Part print with two shaded views. Sizes in mm from the minimum x, y, z corner. A direction names the side the tool comes from. Give positions to 0.01 mm unless a question says otherwise; leave off trailing zeros. Write each loop counter-clockwise with the first axis right and the second up, starting at its lowest first coordinate (ties: lowest second). Pieces come first, ordered by that corner, then holes. Notation, with made-up numbers: M -26.5,17.5 L 6.5,17.5 A33 cw 6.5,56.5 Z; hole C 78,30.25 d1. An arc over 180 degrees is marked long. Return JSON: item names as keys, results as strings. Group by question number.
Q1. Pull direction X, two halves, no side cores. Call the marked faces 1, 2, 3 and 4: +X half, -X half, draft (parallel to the pull), parting line (faces both ways), or undercut.
Q2. Flat gauge pins, fed straight in: pin 1 Ø9.5 at (x, y) = (13.5, 15.5) entering from -Z; pin 2 Ø2 at (x, z) = (12, 21) entering from +Y. Where does each tip first touch, or does it go through?
Q3. Band-saw the part on A-A, the plane z = 5. Give the cut face in (x, y).
Q4. Wall check: probe 1 along Z at (x, y) = (15.25, 3); probe 2 along X at (y, z) = (4.75, 23.5). Give the ranges that are in metal, low to high.
Q5. Tool access for the marked faces 5 and 6: list every direction of +Z, -Z, +X, -X, +Y, -Y with a clear straight run to the whole face (end or side of a thin tool).
Q6. Band-saw the part on C-C, the plane y = 9.25. Give the cut face in (x, z) (3 decimals).
Q7. Band-saw the part on B-B, the plane x = 18.25. Give the cut face in (y, z), then the cut area to 3 significant figures.
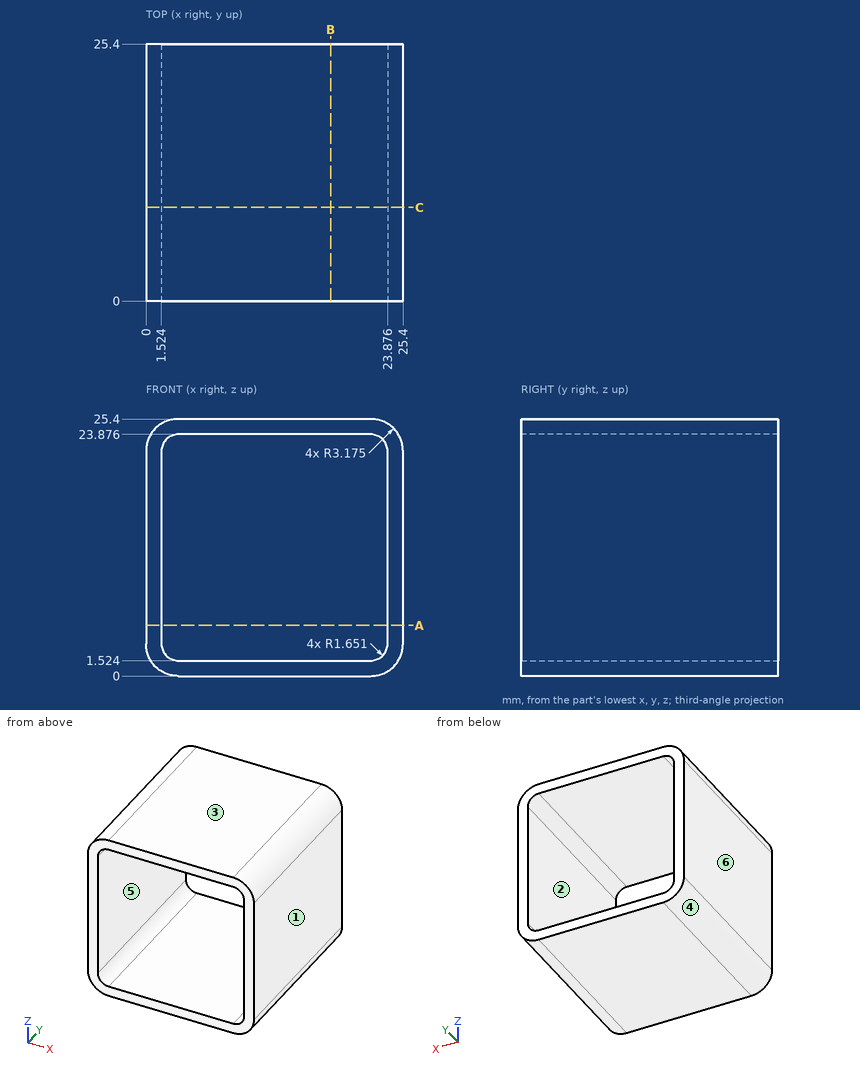
From the geometry:
{
 "1": {"face 1": "+X half", "face 2": "undercut", "face 3": "draft", "face 4": "-X half"},
 "2": {"pin 1": "stops at z = 0", "pin 2": "passes through"},
 "3": {"outline": "M 0,0 L 1.52,0 L 1.52,25.4 L 0,25.4 Z; M 23.88,0 L 25.4,0 L 25.4,25.4 L 23.88,25.4 Z"},
 "4": {"probe 1": "z = 0 to 1.52, 23.88 to 25.4", "probe 2": "x = 0.27 to 2.13, 23.27 to 25.13"},
 "5": {"face 5": "+Y, -Y", "face 6": "+Z, -Z, -X, +Y, -Y"},
 "6": {"outline": "M 0,3.175 A3.175 ccw 3.175,0 L 22.225,0 A3.175 ccw 25.4,3.175 L 25.4,22.225 A3.175 ccw 22.225,25.4 L 3.175,25.4 A3.175 ccw 0,22.225 Z; hole M 1.524,3.175 A1.651 ccw 3.175,1.524 L 22.225,1.524 A1.651 ccw 23.876,3.175 L 23.876,22.225 A1.651 ccw 22.225,23.876 L 3.175,23.876 A1.651 ccw 1.524,22.225 Z"},
 "7": {"outline": "M 0,0 L 25.4,0 L 25.4,1.52 L 0,1.52 Z; M 0,23.88 L 25.4,23.88 L 25.4,25.4 L 0,25.4 Z", "area": "77.4 mm^2"}
}
